```python
from build123d import *

# Parameters (mm, degrees)
F0_W     = 145
F0_H     = 100
F1_DEPTH = 12
F3_DEPTH = 192
F4_W     = 130
F4_H     = 75
F5_DEPTH = 12
F7_D     = 12
F7_DEPTH = 12
F7_TIP   = 3.6051637142
F9_D     = 12
F9_DEPTH = 12
F9_TIP   = 3.6051637142


with BuildPart() as f1:
    # F0 (on Top) → F1 (new body)
    with BuildSketch(Plane.XY):
        with Locations((72.5, 50)):
            Rectangle(F0_W, F0_H)
    extrude(amount=F1_DEPTH)

    # F2 (on face) → F3 (join)
    with BuildSketch(Plane(origin=(0, 0, 0), x_dir=(1, 0, 0), z_dir=(0, 0, -1))):
        with BuildLine():
            ThreePointArc((97.9, -30.95), (96.0401280605, -26.4598719395), (91.55, -24.6))
            Line((91.55, -24.6), (53.45, -24.6))
            ThreePointArc((53.45, -24.6), (48.9598719395, -26.4598719395), (47.1, -30.95))
            Line((47.1, -30.95), (47.1, -69.05))
            ThreePointArc((47.1, -69.05), (48.9598719395, -73.5401280605), (53.45, -75.4))
            Line((53.45, -75.4), (91.55, -75.4))
            ThreePointArc((91.55, -75.4), (96.0401280605, -73.5401280605), (97.9, -69.05))
            Line((97.9, -69.05), (97.9, -30.95))
        make_face()
        with BuildLine():
            Line((56.625, -27.775), (88.375, -27.775))
            ThreePointArc((88.375, -27.775), (92.8651280605, -29.6348719395), (94.725, -34.125))
            Line((94.725, -34.125), (94.725, -65.875))
            ThreePointArc((94.725, -65.875), (92.8651280605, -70.3651280605), (88.375, -72.225))
            Line((88.375, -72.225), (56.625, -72.225))
            ThreePointArc((56.625, -72.225), (52.1348719395, -70.3651280605), (50.275, -65.875))
            Line((50.275, -65.875), (50.275, -34.125))
            ThreePointArc((50.275, -34.125), (52.1348719395, -29.6348719395), (56.625, -27.775))
        make_face(mode=Mode.SUBTRACT)
    extrude(amount=F3_DEPTH)

    # F4 (on face) → F5 (join)
    with BuildSketch(Plane(origin=(0, 0, -192), x_dir=(1, 0, 0), z_dir=(0, 0, -1))):
        with Locations((72.5, -50)):
            Rectangle(F4_W, F4_H)
        with BuildLine():
            ThreePointArc((91.55, -24.6), (96.0401280605, -26.4598719395), (97.9, -30.95))
            Line((97.9, -30.95), (97.9, -69.05))
            ThreePointArc((97.9, -69.05), (96.0401280605, -73.5401280605), (91.55, -75.4))
            Line((91.55, -75.4), (53.45, -75.4))
            ThreePointArc((53.45, -75.4), (48.9598719395, -73.5401280605), (47.1, -69.05))
            Line((47.1, -69.05), (47.1, -30.95))
            ThreePointArc((47.1, -30.95), (48.9598719395, -26.4598719395), (53.45, -24.6))
            Line((53.45, -24.6), (91.55, -24.6))
        make_face(mode=Mode.SUBTRACT)
        with BuildLine():
            Line((97.9, -69.05), (97.9, -30.95))
            ThreePointArc((97.9, -30.95), (96.0401280605, -26.4598719395), (91.55, -24.6))
            Line((91.55, -24.6), (53.45, -24.6))
            ThreePointArc((53.45, -24.6), (48.9598719395, -26.4598719395), (47.1, -30.95))
            Line((47.1, -30.95), (47.1, -69.05))
            ThreePointArc((47.1, -69.05), (48.9598719395, -73.5401280605), (53.45, -75.4))
            Line((53.45, -75.4), (91.55, -75.4))
            ThreePointArc((91.55, -75.4), (96.0401280605, -73.5401280605), (97.9, -69.05))
        make_face()
        with BuildLine():
            ThreePointArc((50.275, -34.125), (52.1348719395, -29.6348719395), (56.625, -27.775))
            Line((56.625, -27.775), (88.375, -27.775))
            ThreePointArc((88.375, -27.775), (92.8651280605, -29.6348719395), (94.725, -34.125))
            Line((94.725, -34.125), (94.725, -65.875))
            ThreePointArc((94.725, -65.875), (92.8651280605, -70.3651280605), (88.375, -72.225))
            Line((88.375, -72.225), (56.625, -72.225))
            ThreePointArc((56.625, -72.225), (52.1348719395, -70.3651280605), (50.275, -65.875))
            Line((50.275, -65.875), (50.275, -34.125))
        make_face(mode=Mode.SUBTRACT)
        with BuildLine():
            Line((88.375, -27.775), (56.625, -27.775))
            ThreePointArc((56.625, -27.775), (52.1348719395, -29.6348719395), (50.275, -34.125))
            Line((50.275, -34.125), (50.275, -65.875))
            ThreePointArc((50.275, -65.875), (52.1348719395, -70.3651280605), (56.625, -72.225))
            Line((56.625, -72.225), (88.375, -72.225))
            ThreePointArc((88.375, -72.225), (92.8651280605, -70.3651280605), (94.725, -65.875))
            Line((94.725, -65.875), (94.725, -34.125))
            ThreePointArc((94.725, -34.125), (92.8651280605, -29.6348719395), (88.375, -27.775))
        make_face()
    extrude(amount=F5_DEPTH)

    # F7 (one way)
    with BuildSketch(Plane.XY.offset(-192)):
        with Locations((122.5, 72.5), (122.5, 27.5), (22.5, 27.5), (22.5, 72.5)):
            Circle(F7_D / 2)
    extrude(amount=-F7_DEPTH, mode=Mode.SUBTRACT)
    with Locations(Plane.XY.offset(-192)):
        with Locations((122.5, 72.5), (122.5, 27.5), (22.5, 27.5), (22.5, 72.5)):
            with Locations((0, 0, -(F7_DEPTH + F7_TIP / 2))):  # 118° drill point
                Cone(0, F7_D / 2, F7_TIP, mode=Mode.SUBTRACT)

    # F9
    with Locations(Plane.XY.offset(12)):
        with Locations((15, 85), (130, 85), (130, 15), (15, 15)):
            Hole(F9_D / 2, depth=F9_DEPTH)
            with Locations((0, 0, -(F9_DEPTH + F9_TIP / 2))):  # 118° drill point
                Cone(0, F9_D / 2, F9_TIP, mode=Mode.SUBTRACT)


solid = f1.part
```
Here's how the part is built. I have some questions about the finished solid (model axes, mm). A direction names the side the tool comes from. Give positions to 0.01 mm unless a question says otherwise; leave off trailing zeros. Loops run counter-clockwise (first coordinate to the right, second up) from the corner with the lowest first, then second, coordinate; pieces in that order, holes last. Notation, with made-up numbers: (2.5, 10) -> (35.5, 10) arc R30 cw to (35.5, 44) -> close; hole circle Ø10 at (41.5, -15.5). An arc over 180 degrees is marked (long way). Use one line per item in the form item = value. Start each with the question number.
1) Imagine slicing it at C-C (z = -66). Please give me the cut outline in (x, y) (3 decimals), then the cut area to 3 significant figures.
2) Please list where these lines run through material, in increasing order: line 1 along X through (y, z) = (85, 9); line 2 along Y through (x, z) = (15, 5.5); line 3 along Z through (x, y) = (64.5, 72).
3) Imagine slicing it at A-A (x = 41). Please give me the cut outline in (y, z).
4) Which directions (+Z, -Z, +X, -X, +Y, -Y) give clear straight access to the entire face, cutting with the end or side of a thin tool? Please do faces 1 (the face through (72, 12.5, -198)), 2 (the face through (137.5, 51, -198)), 3 (the face through (97.9, 50, -95)), 4 (the face through (50.275, 50, -95)), 5 (the face through (47.1, 50, -95)).
5) Imagine slicing it at B-B (y = 15). Please give me the cut outline in (x, z).
6) Thinking about a two-plate mould opening in Y: for faces 6 (the face through (116.506, 27.764, -197.916)), 7 (the face through (145, 49, 6)), 8 (the face through (48.91, 73.49, -94.66)), which applies, +Y half, -Y half, draft (parallel to the pull), parting line (faces both ways), or undercut?
7) For P1, Ø4, axis at x = 57, z = -130, coming from the +Y side; P2, Ø19, axis at y = 55, z = -91.5, coming from the +X side; P3, Ø3, axis at y = 52, z = -17, coming from the -X side, each with a flat end and sliding along its axis, tell me the tip position at first contact or that it passes through.
Check values:
q1.outline = (47.1, 30.95) arc R6.35 ccw to (53.45, 24.6) -> (91.55, 24.6) arc R6.35 ccw to (97.9, 30.95) -> (97.9, 69.05) arc R6.35 ccw to (91.55, 75.4) -> (53.45, 75.4) arc R6.35 ccw to (47.1, 69.05) -> close; hole (50.275, 34.125) arc R6.35 ccw to (56.625, 27.775) -> (88.375, 27.775) arc R6.35 ccw to (94.725, 34.125) -> (94.725, 65.875) arc R6.35 ccw to (88.375, 72.225) -> (56.625, 72.225) arc R6.35 ccw to (50.275, 65.875) -> close
q1.area = 605 mm^2
q2.line_1 = 0 to 9, 21 to 124, 136 to 145
q2.line_2 = 0 to 9, 21 to 79, 91 to 100
q2.line_3 = -204 to -192, 0 to 12
q3.outline = (0, 0) -> (100, 0) -> (100, 12) -> (0, 12) -> close; (12.5, -204) -> (87.5, -204) -> (87.5, -192) -> (12.5, -192) -> close
q4.face_1 = -Z, +X, -X, -Y
q4.face_2 = -Z, +X, +Y, -Y
q4.face_3 = +X, +Y, -Y
q4.face_4 = none
q4.face_5 = -X, +Y, -Y
q5.outline = (0, 0) -> (9, 0) -> (9, 12) -> (0, 12) -> close; (7.5, -204) -> (137.5, -204) -> (137.5, -192) -> (7.5, -192) -> close; (21, 0) -> (124, 0) -> (124, 12) -> (21, 12) -> close; (136, 0) -> (145, 0) -> (145, 12) -> (136, 12) -> close
q6.face_6 = undercut
q6.face_7 = draft
q6.face_8 = +Y half
q7.P1 = 75.4
q7.P2 = 97.9
q7.P3 = 47.1
